Could you check a few things on this model? Use its own coordinates, in mm. Give positions to 0.01 mm unless a question says otherwise; leave off trailing zeros. Order: outer loops, then holes, each group sorted by start corner. A loop starts at its lowest first (then second) coordinate and runs counter-clockwise, first axis right, second up. Notation, with made-up numbers: (-17.5, -15.5) - (41.5, -15.5) arc R25 ccw to (41.5, 4.5) - close; hole circle Ø4 at (-20, 39). An arc over 180 degrees is marked (long way). Put each result on its own line as item: value.
from build123d import *

# Parameters (mm, degrees)
SKETCH1_R           = 2
SKETCH1_R_2         = 1.5
SKETCH1_W           = 3.35
SKETCH1_H           = 30.4
SKETCH1_W_2         = 65
SKETCH1_H_2         = 4
BOSS_EXTRUDE1_DEPTH = 4
FILLET1_R           = 3


with BuildPart() as part:
    # Sketch1 → Boss-Extrude1 (new body)
    with BuildSketch(Plane.XY):
        Polygon((-156.215, 33), (156.215, 33), (156.215, -33), (112.73, -33), (112.73, -37), (-112.73, -37), (-112.73, -33), (-156.215, -33), align=None)
        with Locations((-140.715, 28.5)):
            Circle(SKETCH1_R, mode=Mode.SUBTRACT)
        with Locations((-130.715, 28.5)):
            Circle(SKETCH1_R, mode=Mode.SUBTRACT)
        with Locations((-120.715, 28.5)):
            Circle(SKETCH1_R, mode=Mode.SUBTRACT)
        with Locations((-110.715, 28.5)):
            Circle(SKETCH1_R, mode=Mode.SUBTRACT)
        with Locations((-100.715, 28.5)):
            Circle(SKETCH1_R, mode=Mode.SUBTRACT)
        with Locations((-57.595, 28.5)):
            Circle(SKETCH1_R, mode=Mode.SUBTRACT)
        with Locations(Location((57.595, 28.5, 0), (0, 0, 180))):
            Circle(SKETCH1_R, mode=Mode.SUBTRACT)
        with Locations(Location((100.715, 28.5, 0), (0, 0, 180))):
            Circle(SKETCH1_R, mode=Mode.SUBTRACT)
        with Locations(Location((110.715, 28.5, 0), (0, 0, 180))):
            Circle(SKETCH1_R, mode=Mode.SUBTRACT)
        with Locations(Location((120.715, 28.5, 0), (0, 0, 180))):
            Circle(SKETCH1_R, mode=Mode.SUBTRACT)
        with Locations(Location((130.715, 28.5, 0), (0, 0, 180))):
            Circle(SKETCH1_R, mode=Mode.SUBTRACT)
        with Locations(Location((140.715, 28.5, 0), (0, 0, 180))):
            Circle(SKETCH1_R, mode=Mode.SUBTRACT)
        with Locations((-140.715, -25)):
            Circle(SKETCH1_R, mode=Mode.SUBTRACT)
        with Locations((-130.715, -25)):
            Circle(SKETCH1_R, mode=Mode.SUBTRACT)
        with Locations((-120.715, -25)):
            Circle(SKETCH1_R, mode=Mode.SUBTRACT)
        with Locations((-110.715, -25)):
            Circle(SKETCH1_R, mode=Mode.SUBTRACT)
        with Locations((-100.715, -25)):
            Circle(SKETCH1_R, mode=Mode.SUBTRACT)
        with Locations((-57.595, -25)):
            Circle(SKETCH1_R, mode=Mode.SUBTRACT)
        with Locations(Location((140.715, -25, 0), (0, 0, 180))):
            Circle(SKETCH1_R, mode=Mode.SUBTRACT)
        with Locations(Location((130.715, -25, 0), (0, 0, 180))):
            Circle(SKETCH1_R, mode=Mode.SUBTRACT)
        with Locations(Location((120.715, -25, 0), (0, 0, 180))):
            Circle(SKETCH1_R, mode=Mode.SUBTRACT)
        with Locations(Location((110.715, -25, 0), (0, 0, 180))):
            Circle(SKETCH1_R, mode=Mode.SUBTRACT)
        with Locations(Location((100.715, -25, 0), (0, 0, 180))):
            Circle(SKETCH1_R, mode=Mode.SUBTRACT)
        with Locations(Location((57.595, -25, 0), (0, 0, 180))):
            Circle(SKETCH1_R, mode=Mode.SUBTRACT)
        with Locations((3.565, -24)):
            Circle(SKETCH1_R_2, mode=Mode.SUBTRACT)
        with Locations((3.565, 20)):
            Circle(SKETCH1_R_2, mode=Mode.SUBTRACT)
        with Locations((87.565, 20)):
            Circle(SKETCH1_R_2, mode=Mode.SUBTRACT)
        with Locations((87.565, -24)):
            Circle(SKETCH1_R_2, mode=Mode.SUBTRACT)
        with Locations((150.74, -1.98)):
            Rectangle(SKETCH1_W, SKETCH1_H, mode=Mode.SUBTRACT)
        with Locations((-150.74, -1.98)):
            Rectangle(SKETCH1_W, SKETCH1_H, mode=Mode.SUBTRACT)
        with Locations((-0.085, -31)):
            Rectangle(SKETCH1_W_2, SKETCH1_H_2, mode=Mode.SUBTRACT)
    extrude(amount=BOSS_EXTRUDE1_DEPTH)

    # Fillet1
    fillet1_edges = [part.edges().sort_by_distance(p)[0] for p in [
        (112.73, -37, 2),
        (-112.73, -37, 2),
        (-156.215, -33, 2),
        (-156.215, 33, 2),
        (156.215, 33, 2),
        (156.215, -33, 2),
    ]]
    fillet(fillet1_edges, radius=FILLET1_R)


solid = part.part
1) I'm going to push a flat-ended pin straight in: pin 1 (1.7 mm diameter, centred on x = 150, z = 2, fed in from -Y). Where does the tip first touch, or does it pass through?
Filled in:
pin 1: stops at y = -33
2) Suppose I cut it at A-A, the plane y = -0.5. List the corners of the cut face in (x, z) for me (3 decimals), and give its area (3 significant figures).
Filled in:
outline: (-156.215, 0) - (-152.415, 0) - (-152.415, 4) - (-156.215, 4) - close; (-149.065, 0) - (149.065, 0) - (149.065, 4) - (-149.065, 4) - close; (152.415, 0) - (156.215, 0) - (156.215, 4) - (152.415, 4) - close
area: 1,220 mm^2
3) Suppose I cut it at B-B, the plane z = 2.65. State how many separate pieces and enclosed holes the cut face has, and give its area (3 significant figures).
Filled in:
separate pieces: 1
enclosed holes: 31
area: 20,700 mm^2
4) If I drill on line 1 (X direction, y = 1.5, z = 3.25) (3 decimals); line 2 (Y direction, x = -140.5, z = 3.65); line 3 (Y direction, x = 8, z = 1.25), over which ranges is the centre line in solid material (lowest first)? Write a range as [from, to].
Filled in:
line 1: x = [-156.215, -152.415], [-149.065, 149.065], [152.415, 156.215]
line 2: y = [-33, -26.99], [-23.01, 26.51], [30.49, 33]
line 3: y = [-37, -33], [-29, 33]
